The listing builds one solid part. Answer for the finished solid, in the listing's coordinates (mm). Face numbers are marked on the shaded views. A direction names the side the tool comes from. Round coordinates to 2 decimals unless told otherwise and drop trailing zeros. Write each loop counter-clockwise with the first axis right and the second up, starting at its lowest first coordinate (ties: lowest second). Pieces come first, ordered by that corner, then holes. Notation, with made-up numbers: (33.5, -7) - (61.5, -7) arc R29 ccw to (61.5, 25) - close; hole circle Ø11 at (4, 52.25). An arc over 180 degrees is marked (long way). Answer as CSV lines item,"result". Start each with the question number.
Item 1: Flat-ended cylindrical pins translate along their axes: pin 1 (3 mm diameter, centred on y = 41.5, z = 12.5, fed in from +X); pin 2 (3 mm diameter, centred on x = 53.5, y = 61, fed in from -Z). Find the tip coordinate at first contact, or state that the pin passes through.
Item 2: Which of the six approach directions +Z, -Z, +X, -X, +Y, -Y give full straight-line access (tool end or side, diameter ignored) to the marked faces 4 and 5?
Item 3: Straight lines are drawn through the part: line 1 along Y through (x, z) = (64, 48); line 2 along X through (y, z) = (50, 10.5); line 3 along Z through (x, y) = (57, 58). For each, find the intervals that lie inside material, in ascending order. Write a range as [from, to].
Item 4: A cutting plane is placed at C-C on z = 25.5. Determine the outline of the cut face in (x, y), and give its area (3 significant figures).
Item 5: For a pull along Y with two mould halves and no side action, classify the marked faces 1, 2 and 3 as pulls with the +Y half, pulls with the -Y half, needs draft (parallel to the pull), parting line crosses it, or undercut.
Item 6: A cutting plane is placed at A-A on z = 4. Determine the outline of the cut face in (x, y), and give its area (3 significant figures).
Item 7: A cutting plane is placed at B-B on y = 80.5. Determine the outline of the cut face in (x, z).
Item 8: A cutting plane is placed at D-D on y = 42.5. Determine the outline of the cut face in (x, z), and give its area (4 significant figures).
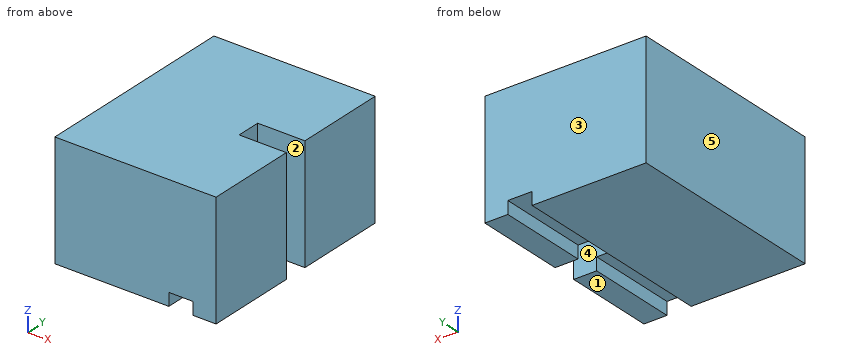
```python
from build123d import *

# Parameters (mm, degrees)
SKICA1_W                      = 70
SKICA1_H                      = 90
P_IDAT_VYSUNUT_M1_DEPTH       = 50
SKICA7_W                      = 20.5
SKICA7_H                      = 10.5
ODEBRAT_VYSUNUT_M3_DEPTH      = 50
ODEBRAT_VYSUNUT_M4_DEPTH      = 60
ODEBRAT_VYSUNUT_M4_DEPTH_BACK = 50
SKICA9_W                      = 10.5
SKICA9_H                      = 5.5


with BuildPart() as part:
    # Skica1 → Přidat vysunutím1 (new body)
    with BuildSketch(Plane.XY):
        with Locations((35, 45)):
            Rectangle(SKICA1_W, SKICA1_H)
    extrude(amount=P_IDAT_VYSUNUT_M1_DEPTH)

    # Skica7 → Odebrat vysunutím3 (cut)
    with BuildSketch(Plane(origin=(0, 0, 0), x_dir=(-1, 0, 0), z_dir=(0, 0, -1))):
        with Locations((-59.75, 45)):
            Rectangle(SKICA7_W, SKICA7_H)
    extrude(amount=-ODEBRAT_VYSUNUT_M3_DEPTH, mode=Mode.SUBTRACT)

    # Skica9 → Odebrat vysunutím4 (cut, two sides: drawn at the far end of the back side and taken through both)
    with BuildSketch(Plane.XZ.offset(-50.25).offset(-ODEBRAT_VYSUNUT_M4_DEPTH_BACK)):
        with Locations((54.75, 2.75)):
            Rectangle(SKICA9_W, SKICA9_H)
    extrude(amount=ODEBRAT_VYSUNUT_M4_DEPTH + ODEBRAT_VYSUNUT_M4_DEPTH_BACK, mode=Mode.SUBTRACT)


solid = part.part
```
Geometry says:
1,pin 1,"stops at x = 49.5"
1,pin 2,"stops at z = 5.5"
2,face 4,"+Z, -Z, +X"
2,face 5,"+Z, -Z, -X, +Y, -Y"
3,line 1,"y = [0, 39.75], [50.25, 90]"
3,line 2,"x = [0, 49.5]"
3,line 3,"z = [5.5, 50]"
4,outline,"(0, 0) - (70, 0) - (70, 39.75) - (49.5, 39.75) - (49.5, 50.25) - (70, 50.25) - (70, 90) - (0, 90) - close"
4,area,"6,080 mm^2"
5,face 1,"needs draft"
5,face 2,"undercut"
5,face 3,"pulls with the +Y half"
6,outline,"(0, 0) - (49.5, 0) - (49.5, 90) - (0, 90) - close; (60, 0) - (70, 0) - (70, 39.75) - (60, 39.75) - close; (60, 50.25) - (70, 50.25) - (70, 90) - (60, 90) - close"
6,area,"5,250 mm^2"
7,outline,"(0, 0) - (49.5, 0) - (49.5, 5.5) - (60, 5.5) - (60, 0) - (70, 0) - (70, 50) - (0, 50) - close"
8,outline,"(0, 0) - (49.5, 0) - (49.5, 50) - (0, 50) - close"
8,area,"2,475 mm^2"
